The model under review builds one solid part; all positions refer to its coordinate system, in mm. A direction names the side the tool comes from. Round coordinates to 2 decimals unless told otherwise and drop trailing zeros. Loops run counter-clockwise (first coordinate to the right, second up) from the corner with the lowest first, then second, coordinate; pieces in that order, holes last. Notation, with made-up numbers: M -27.5,-8 L -21.5,-8 A13 cw -21.5,0 Z; hole C 28.5,4 d1. An arc over 180 degrees is marked long. One line per question, with ' | ' between items.
from build123d import *

# Parameters (mm, degrees)
F1_DEPTH = 9.525
F3_D     = 3.175
F5_D     = 3.175


# Not quite as in the source:
# - ends of sketch curves that miss each other by under 0.0002 mm in the source are joined
# - a length typed as a fraction of an inch, garbled in the dataset ("3 / 203.2 mm" for 3/8 in), is restored


with BuildPart() as f1:
    # F0 (on Top) → F1 (new body)
    with BuildSketch(Plane.XY):
        with BuildLine():
            ThreePointArc((7.6885502785, 1.9437116954), (5.4434862483, 1.0137757257), (4.5135502785, -1.2312883046))
            Line((4.5135502785, -1.2312883046), (6.1010502795, -1.2312883046))
            ThreePointArc((6.1010502795, -1.2312883046), (7.6885771705, 0.3561579113), (9.2760502785, -1.2313420884))
            Line((9.2760502785, -1.2313420884), (10.8635502785, -1.2312883046))
            ThreePointArc((10.8635502785, -1.2312883046), (9.9336143088, 1.0137757257), (7.6885502785, 1.9437116954))
        make_face()
        with BuildLine():
            Line((-5.0114497215, -1.2312883046), (-5.0114497215, -4.4062883046))
            Line((-5.0114497215, -4.4062883046), (20.3885502785, -4.4062883046))
            Line((20.3885502785, -4.4062883046), (20.3885502785, -1.2312883046))
            Line((20.3885502785, -1.2312883046), (10.8635502785, -1.2312883046))
            Line((10.8635502785, -1.2312883046), (9.2760502785, -1.2312883046))
            ThreePointArc((9.2760502785, -1.2312883046), (7.6885233866, -2.8188420882), (6.1010502795, -1.2312883046))
            Line((6.1010502795, -1.2312883046), (4.5135502785, -1.2312883046))
            Line((4.5135502785, -1.2312883046), (-5.0114497215, -1.2312883046))
        make_face()
    extrude(amount=F1_DEPTH)

    # F3 (through all)
    with Locations(Plane(origin=(0, -1.2312883046, 0), x_dir=(-1, 0, 0), z_dir=(0, 1, 0))):
        with Locations((-15.6260502785, 4.7625)):
            Hole(F3_D / 2)

    # F5 (through all)
    with Locations(Plane(origin=(0, -1.2312883046, 0), x_dir=(-1, 0, 0), z_dir=(0, 1, 0))):
        with Locations((0.2489497215, 4.7625)):
            Hole(F5_D / 2)


solid = f1.part
1) Add section C-C on z = 5.5. State how many separate pieces and enclosed holes the cut face has, then the cut area to 3 significant figures.
Output values:
separate pieces: 3 | enclosed holes: 1 | area: 70.7 mm²
2) Insertion check: P1, Ø2, axis at y = 0, z = 3, coming from the -X side; P2, Ø5, axis at x = 15.63, z = 4.76, coming from the +Y side. Each pin has a flat end and moves straight along its axis. Give the tip position at first contact, or say it passes through.
Output values:
P1: stops at x = 4.52 | P2: stops at y = -1.23
3) Mouldability with a two-part tool opening along Z and no side actions: class faces 4 (the cylindrical face through (0.604, -2.841, 6.101)), 5 (the flat face through (-5.011, -3, 5)), 6 (the flat face through (8, -3, 0)) as +Z half, -Z half, draft (parallel to the pull), parting line (faces both ways), or undercut.
Output values:
face 4: undercut | face 5: draft | face 6: -Z half
4) Machinability: for faces 1 (the flat face through (20.389, -3, 5)), 2 (the flat face through (18, -1.231, 5)), 3 (the flat face through (2, -1.231, 5)), which of the approach directions +Z, -Z, +X, -X, +Y, -Y give a long, thin tool a straight path to every point of the face, cutting with its end or side? Answer none if there is none.
Output values:
face 1: +Z, -Z, +X, +Y, -Y | face 2: +Z, -Z, +X, +Y | face 3: +Z, -Z, -X, +Y
5) Add section D-D on x = 8. State the section outline as (y, z) points (3 decimals).
Output values:
outline: M -4.406,0 L -2.788,0 L -2.788,9.525 L -4.406,9.525 Z; M 0.325,0 L 1.928,0 L 1.928,9.525 L 0.325,9.525 Z
6) For line 1 (X direction, y = -3.5, z = 5.25); line 2 (X direction, y = -4, z = 4.5); line 3 (Y direction, x = 15.75, z = 8), list the stretches that pass through material, from the lowest coordinate up.
Output values:
line 1: x = -5.01 to -1.76, 1.26 to 14.12, 17.14 to 20.39 | line 2: x = -5.01 to -1.81, 1.32 to 14.06, 17.19 to 20.39 | line 3: y = -4.41 to -1.23
7) Add section B-B on y = -2. State the section outline as (x, z) points (1 decimal), then the cut area to 3 significant figures.
Output values:
outline: M -5,0 L 6.3,0 L 6.3,9.5 L -5,9.5 Z; M 9.1,0 L 20.4,0 L 20.4,9.5 L 9.1,9.5 Z; hole C -0.2,4.8 d3.2; hole C 15.6,4.8 d3.2 | area: 200 mm²
